Design review of the part shown in the three views and the two pictorial views. Dimensions are in mm from the part's minimum x, y and z. A direction names the side the tool comes from. Round coordinates to 2 decimals unless told otherwise and drop trailing zeros. Loops run counter-clockwise (first coordinate to the right, second up) from the corner with the lowest first, then second, coordinate; pieces in that order, holes last. Notation, with made-up numbers: (-31.5, 65) - (-21.5, 65) arc R27 cw to (-21.5, 101) - close; hole circle Ø2 at (-13, 24.5). An arc over 180 degrees is marked (long way). Return JSON: item names as keys, results as strings. Group by question number.
(1) Wall thickness on L1, parallel to X at y = 76, z = 36; L2, parallel to Z at x = 66, y = 23.5: over which ranges is each line inside the solid? List them lowest first. Write a range as [from, to].
(2) Clearance check with a flat-ended pin moving along its axis: pin 1 (10 mm diameter, centred on x = 48.5, y = 19, fed in from +Z). State where the tip first meets the part, or that it passes through.
(3) For the marked faces 4 and 5, list the 3-axis set-ups (+Z, -Z, +X, -X, +Y, -Y) from which the entire face can be reached by the end or side of a thin tool; tool diameter is ignored.
(4) We need section D-D, the plane z = 61.5. Write out the cut boundary in (x, y).
(5) We need section C-C, the plane y = 77.5. Write out the cut boundary in (x, z).
(6) The part is to be moulded in two halves that separate along Y. For the marked faces 1, 2 and 3, say which applies: pulls with the +Y half, pulls with the -Y half, needs draft (parallel to the pull), parting line crosses it, or undercut.
(7) We need section B-B, the plane z = 93. Write out the cut boundary in (x, y).
(8) We need section A-A, the plane y = 46.5. Write out the cut boundary in (x, z), and give its area (4 significant figures).
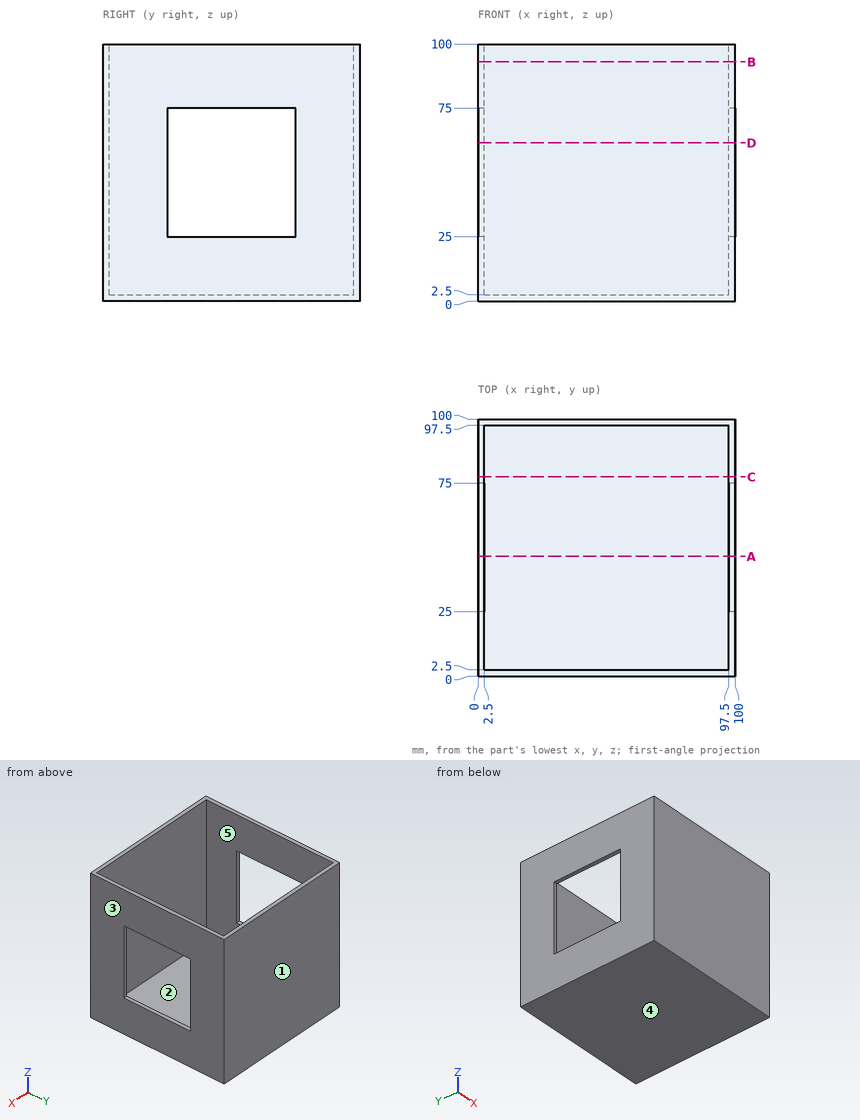
Solutions:
{
 "1": {"L1": "[0, 2.5], [97.5, 100]", "L2": "[0, 2.5]"},
 "2": {"pin 1": "z = 2.5"},
 "3": {"face 4": "-Z, +X, -X, +Y, -Y", "face 5": "+Z"},
 "4": {"outline": "(0, 0) - (100, 0) - (100, 25) - (97.5, 25) - (97.5, 2.5) - (2.5, 2.5) - (2.5, 25) - (0, 25) - close; (0, 75) - (2.5, 75) - (2.5, 97.5) - (97.5, 97.5) - (97.5, 75) - (100, 75) - (100, 100) - (0, 100) - close"},
 "5": {"outline": "(0, 0) - (100, 0) - (100, 100) - (97.5, 100) - (97.5, 2.5) - (2.5, 2.5) - (2.5, 100) - (0, 100) - close"},
 "6": {"face 1": "pulls with the +Y half", "face 2": "undercut", "face 3": "needs draft"},
 "7": {"outline": "(0, 0) - (100, 0) - (100, 100) - (0, 100) - close; hole (2.5, 2.5) - (97.5, 2.5) - (97.5, 97.5) - (2.5, 97.5) - close"},
 "8": {"outline": "(0, 0) - (100, 0) - (100, 25) - (97.5, 25) - (97.5, 2.5) - (2.5, 2.5) - (2.5, 25) - (0, 25) - close; (0, 75) - (2.5, 75) - (2.5, 100) - (0, 100) - close; (97.5, 75) - (100, 75) - (100, 100) - (97.5, 100) - close", "area": "487.5 mm^2"}
}
